```python
from build123d import *

# Parameters (mm, degrees)
F0_R     = 62.3719654877
F1_DEPTH = 3.5956986248
F3_SIZE  = 5.08


# Not quite as in the source:
# - a fillet or chamfer that OpenCascade refuses, or shapes differently, is made with other operations: its cross-section is extruded or revolved along the edge and cut away or added


with BuildPart() as f1:
    # F0 (on Front) → F1 (new body)
    with BuildSketch(Plane.XZ):
        with Locations((-8.0392340643, 1.049432549)):
            Circle(F0_R)
    extrude(amount=-F1_DEPTH)

    # F2: chamfer of 5.08 on 1 edges, made by hand

    # F2_s1 → F2_t2 (revolve, cut)
    with BuildSketch(Plane.XY.offset(1.049432549)):
        Polygon((54.3327314234, 5.08), (49.2527314234, 0), (54.3327314234, 0), align=None)
    revolve(axis=Axis((-8.0392340643, 0, 1.049432549), (0, -1, 0)), mode=Mode.SUBTRACT)

    # F3
    f3_edges = [f1.edges().sort_by_distance(p)[0] for p in [
        (-68.926898, 3.595699, 1.049433),
    ]]
    chamfer(f3_edges, length=F3_SIZE)


solid = f1.part
```
For this review, take the finished solid that the model builds, in its own axes (mm). Round coordinates to 2 decimals unless told otherwise and drop trailing zeros. Loops run counter-clockwise (first coordinate to the right, second up) from the corner with the lowest first, then second, coordinate; pieces in that order, holes last.
Q1. Add section A-A on y = 2.15. Write out the cut boundary in (x, z).
Result sheet:
outline: circle Ø112.81 at (-8.04, 1.05)
Q2. Insertion check: pin 1 Ø1 at (x, y) = (-32.5, 1.5) entering from -Z; pin 2 Ø1.5 at (y, z) = (2.5, -21) entering from +X; pin 3 Ø1 at (y, z) = (1.5, -38) entering from -X. Each pin has a flat end and moves straight along its axis. Give the tip position at first contact, or say it passes through.
Result sheet:
pin 1: stops at z = -50.41
pin 2: stops at x = 44.18
pin 3: stops at x = -49.66
Q3. To check wall thickness, follow line 1 along X through (y, z) = (2.45, 50); line 2 along X through (y, z) = (2, -47); line 3 along Z through (x, y) = (19, 0.35). State the ranges of each line that lie inside material, in increasing order.
Result sheet:
line 1: x = -35.82 to 19.74
line 2: x = -37.7 to 21.62
line 3: z = -49.3 to 51.4
